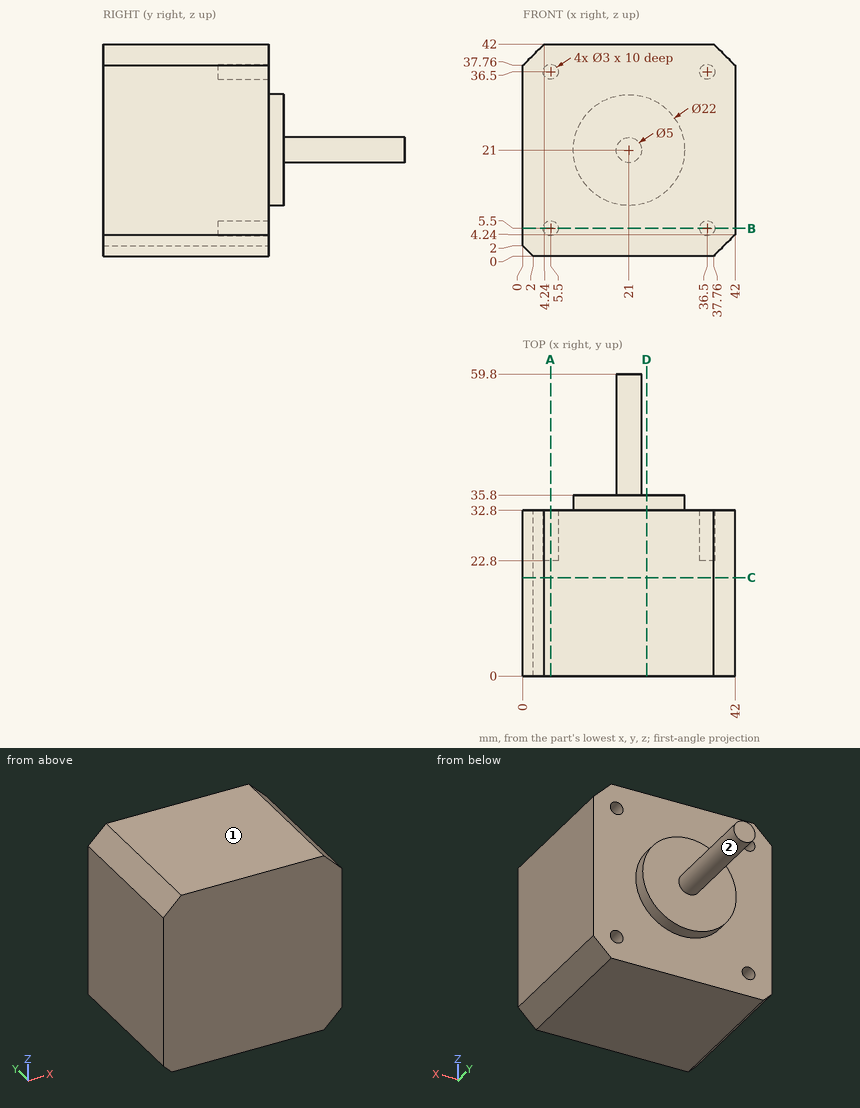
Part print with two shaded views. Sizes in mm from the minimum x, y, z corner. A direction names the side the tool comes from. Coordinates: 2 decimals unless noted, no trailing zeros. Write each loop counter-clockwise with the first axis right and the second up, starting at its lowest first coordinate (ties: lowest second). Pieces come first, ordered by that corner, then holes. Notation, with made-up numbers: (4.5, 60.25) -> (19.5, 60.25) arc R28 cw to (19.5, 85.25) -> close; hole circle Ø5 at (36, 51.5). An arc over 180 degrees is marked (long way). Return JSON: item names as keys, results as strings. Group by question number.
Q1. Cut at D-D, the plane x = 24.5. Give the cut face in (y, z).
Q2. Drill centre lines: line 1 (Z direction, x = 5.5, y = 27.75); line 2 (Y direction, x = 40, z = 18.5). Where is each one in solid material? Low to high.
Q3. Cut at A-A, the plane x = 5.5. Give the cut face in (y, z), then the cut area to 3 significant figures.
Q4. Cut at C-C, the plane y = 19.5. Give the cut face in (x, z), then the cut area to 3 significant figures.
Q5. Cut at B-B, the plane z = 5.5. Give the cut face in (x, y), then the cut area to 3 significant figures.
Q6. Flat gauge pins, fed straight in: pin 1 (0.9 mm diameter, centred on x = 36.5, z = 5, fed in from +Y); pin 2 (3.5 mm diameter, centred on x = 36.5, z = 5.5, fed in from +Y); pin 3 (8 mm diameter, centred on x = 13, y = 49, fed in from -Z). Where does each tip first touch, or does it go through?
Q7. Which spindle directions (+Z, -Z, +X, -X, +Y, -Y) get a long thin tool onto all of the face, cutting with end or side? Do the marked faces 1 and 2. Say none if no direction does.
Returned:
{
 "1": {"outline": "(0, 0) -> (32.8, 0) -> (32.8, 10.57) -> (35.8, 10.57) -> (35.8, 31.43) -> (32.8, 31.43) -> (32.8, 42) -> (0, 42) -> close"},
 "2": {"line 1": "z = 0 to 4, 7 to 35, 38 to 42", "line 2": "y = 0 to 32.8"},
 "3": {"outline": "(0, 0) -> (32.8, 0) -> (32.8, 4) -> (22.8, 4) -> (22.8, 7) -> (32.8, 7) -> (32.8, 35) -> (22.8, 35) -> (22.8, 38) -> (32.8, 38) -> (32.8, 42) -> (0, 42) -> close", "area": "1,320 mm2"},
 "4": {"outline": "(0, 2) -> (2, 0) -> (37.76, 0) -> (42, 4.24) -> (42, 37.76) -> (37.76, 42) -> (4.24, 42) -> (0, 37.76) -> close", "area": "1,740 mm2"},
 "5": {"outline": "(0, 0) -> (42, 0) -> (42, 32.8) -> (38, 32.8) -> (38, 22.8) -> (35, 22.8) -> (35, 32.8) -> (7, 32.8) -> (7, 22.8) -> (4, 22.8) -> (4, 32.8) -> (0, 32.8) -> close", "area": "1,320 mm2"},
 "6": {"pin 1": "stops at y = 22.8", "pin 2": "stops at y = 32.8", "pin 3": "passes through"},
 "7": {"face 1": "+Z, +X, -X, +Y, -Y", "face 2": "+Y"}
}
